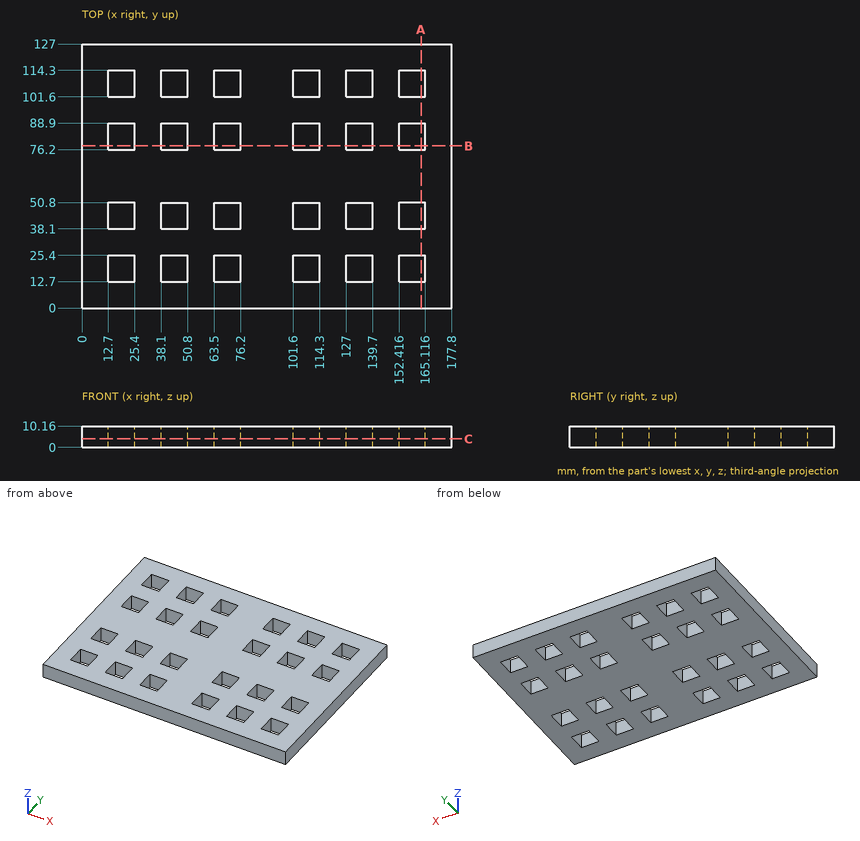
Job drawing, mm, ordinate dimensions from the low corner. One solid piece. Coordinates: 2 decimals unless noted, no trailing zeros. Loops run counter-clockwise (first coordinate to the right, second up) from the corner with the lowest first, then second, coordinate; pieces in that order, holes last. Notation, with made-up numbers: (40.25, 76.25) - (64.25, 76.25) arc R34 cw to (64.25, 107.25) - close; hole circle Ø2 at (30.5, 10). An arc over 180 degrees is marked (long way). Write item = value, one per line. Start each with the question number.
Q1. Cut at B-B, the plane y = 78. List the corners of the cut face in (x, z) (1 decimal).
Q2. Cut at A-A, the plane x = 163. List the corners of the cut face in (y, z).
Q3. Cut at C-C, the plane z = 4. Give the number of separate pieces and of enclosed holes in the cut face, then the cut area to 3 significant figures.
Q4. Flat gauge pin, fed straight in: pin 1 Ø1.5 at (x, y) = (74, 110) entering from +Z. Where does the tip first touch, or does it go through?
Q5. Drill centre line: L1, parallel to Y at x = 50, z = 1.5. Where is it in solid material? Low to high.
Computed:
q1.outline = (0, 0) - (12.7, 0) - (12.7, 10.2) - (0, 10.2) - close; (25.4, 0) - (38.1, 0) - (38.1, 10.2) - (25.4, 10.2) - close; (50.8, 0) - (63.5, 0) - (63.5, 10.2) - (50.8, 10.2) - close; (76.2, 0) - (101.6, 0) - (101.6, 10.2) - (76.2, 10.2) - close; (114.3, 0) - (127, 0) - (127, 10.2) - (114.3, 10.2) - close; (139.7, 0) - (152.4, 0) - (152.4, 10.2) - (139.7, 10.2) - close; (165.1, 0) - (177.8, 0) - (177.8, 10.2) - (165.1, 10.2) - close
q2.outline = (0, 0) - (12.7, 0) - (12.7, 10.16) - (0, 10.16) - close; (25.4, 0) - (38.1, 0) - (38.1, 10.16) - (25.4, 10.16) - close; (50.8, 0) - (76.2, 0) - (76.2, 10.16) - (50.8, 10.16) - close; (88.9, 0) - (101.6, 0) - (101.6, 10.16) - (88.9, 10.16) - close; (114.3, 0) - (127, 0) - (127, 10.16) - (114.3, 10.16) - close
q3.separate_pieces = 1
q3.enclosed_holes = 24
q3.area = 18,700 mm²
q4.pin_1 = through
q5.L1 = 0 to 12.7, 25.4 to 38.1, 50.8 to 76.2, 88.9 to 101.6, 114.3 to 127
